from build123d import *

# Parameters (mm, degrees)
SKETCH1_W           = 30
SKETCH1_H           = 30
BOSS_EXTRUDE1_DEPTH = 3.1
SKETCH2_W           = 3.1
SKETCH2_H           = 3.1
CUT_EXTRUDE1_DEPTH  = 15
FILLET1_R           = 5


with BuildPart() as part:
    # Sketch1 → Boss-Extrude1 (new body)
    with BuildSketch(Plane.XY):
        Rectangle(SKETCH1_W, SKETCH1_H)
    extrude(amount=BOSS_EXTRUDE1_DEPTH)

    # Sketch2 → Cut-Extrude1 (cut)
    with BuildSketch(Plane(origin=(0, 15, 0), x_dir=(1, 0, 0), z_dir=(0, 1, 0))):
        with Locations((0, -1.55)):
            Rectangle(SKETCH2_W, SKETCH2_H)
    extrude(amount=-CUT_EXTRUDE1_DEPTH, mode=Mode.SUBTRACT)

    # Fillet1
    fillet1_edges = [part.edges().sort_by_distance(p)[0] for p in [
        (15, -15, 1.55),
        (-15, -15, 1.55),
        (-15, 15, 1.55),
        (15, 15, 1.55),
    ]]
    fillet(fillet1_edges, radius=FILLET1_R)


solid = part.part
Read the model definition and answer for the solid it produces. Units are mm, in the model's axes. A direction names the side the tool comes from. Round coordinates to 2 decimals unless told otherwise and drop trailing zeros. Write each loop counter-clockwise with the first axis right and the second up, starting at its lowest first coordinate (ties: lowest second). Pieces come first, ordered by that corner, then holes.
1. Straight lines are drawn through the part: L1, parallel to X at y = 3.75, z = 2.4; L2, parallel to X at y = -10.25, z = 1.3; L3, parallel to Y at x = -0.25, z = 1.3. For each, find the intervals that lie inside material, in ascending order.
2. The part is cut by section A-A, the plane y = 8. Determine the outline of the cut face in (x, z), then the cut area to 3 significant figures.
3. The part is cut by section D-D, the plane x = -13. Determine the outline of the cut face in (y, z).
4. Which of the six approach directions +Z, -Z, +X, -X, +Y, -Y give full straight-line access (tool end or side, diameter ignored) to faces 1 (the face through (-1.55, 8, 2)), 2 (the face through (-14, 13, 2))?
5. Determine the mould class of faces 3 (the face through (0, -15, 2)), 4 (the face through (1.55, 8, 2)), 5 (the face through (13, -14, 2)) for opening direction X: pulls with the +X half, pulls with the -X half, needs draft (parallel to the pull), parting line crosses it, or undercut.
6. The part is cut by section C-C, the plane x = -0.75. Determine the outline of the cut face in (y, z), then the cut area to 3 significant figures.
7. Given pin 1 Ø1.6 at (x, z) = (-0.5, 1.5) entering from +Y; pin 2 Ø8 at (x, y) = (-5.5, 8.5) entering from -Z, each flat-ended and moving along its own axis, determine where each tip first touches the part or whether it passes through.
8. The part is cut by section B-B, the plane z = 0.95. Determine the outline of the cut face in (x, y).
Values:
1. L1: x = -15 to -1.55, 1.55 to 15
1. L2: x = -14.99 to 14.99
1. L3: y = -15 to 0
2. outline: (-15, 0) - (-1.55, 0) - (-1.55, 3.1) - (-15, 3.1) - close; (1.55, 0) - (15, 0) - (15, 3.1) - (1.55, 3.1) - close
2. area: 83.4 mm2
3. outline: (-14, 0) - (14, 0) - (14, 3.1) - (-14, 3.1) - close
4. face 1: +Z, -Z, +Y
4. face 2: +Z, -Z, -X, +Y
5. face 3: needs draft
5. face 4: undercut
5. face 5: pulls with the +X half
6. outline: (-15, 0) - (0, 0) - (0, 3.1) - (-15, 3.1) - close
6. area: 46.5 mm2
7. pin 1: stops at y = 0
7. pin 2: stops at z = 0
8. outline: (-15, -10) arc R5 ccw to (-10, -15) - (10, -15) arc R5 ccw to (15, -10) - (15, 10) arc R5 ccw to (10, 15) - (1.55, 15) - (1.55, 0) - (-1.55, 0) - (-1.55, 15) - (-10, 15) arc R5 ccw to (-15, 10) - close
